Verification items for the finished model (mm, model axes). A direction names the side the tool comes from. Coordinates: 2 decimals unless noted, no trailing zeros. Write each loop counter-clockwise with the first axis right and the second up, starting at its lowest first coordinate (ties: lowest second). Pieces come first, ordered by that corner, then holes. Notation, with made-up numbers: (81, 38.25) -> (137, 38.25) arc R17 ccw to (137, 64.25) -> close; hole circle Ø7 at (8, 13). An arc over 180 degrees is marked (long way). Use a Markdown table: item, result. Add a question column.
from build123d import *

# Parameters (mm, degrees)
F0_R     = 14
F1_DEPTH = 40
F2_R     = 5.5
F3_DEPTH = 15
F2_R_2   = 9
F4_DEPTH = 7.3


with BuildPart() as f1:
    # F0 (on Front) → F1 (new body)
    with BuildSketch(Plane.XZ):
        with BuildLine():
            Line((-55, 0), (0, 0))
            Line((0, 0), (55, 0))
            Line((55, 0), (55, 15))
            Line((55, 15), (25, 15))
            Line((25, 15), (25, 40))
            ThreePointArc((25, 40), (0, 66), (-25, 40))
            Line((-25, 40), (-25, 15))
            Line((-25, 15), (-55, 15))
            Line((-55, 15), (-55, 0))
        make_face()
        with Locations((0, 40)):
            Circle(F0_R, mode=Mode.SUBTRACT)
    extrude(amount=F1_DEPTH)

    # F2 (on face) → F3 (cut)
    with BuildSketch(Plane.XY.offset(15)):
        with Locations((40, -20)):
            Circle(F2_R)
        with Locations((-40, -20)):
            Circle(F2_R)
    extrude(amount=-F3_DEPTH, mode=Mode.SUBTRACT)

    # F2 (on face) → F4 (cut)
    with BuildSketch(Plane.XY.offset(15)):
        with Locations((40, -20)):
            Circle(F2_R_2)
        with Locations((40, -20)):
            Circle(F2_R, mode=Mode.SUBTRACT)
        with Locations((-40, -20)):
            Circle(F2_R_2)
        with Locations((-40, -20)):
            Circle(F2_R, mode=Mode.SUBTRACT)
    extrude(amount=-F4_DEPTH, mode=Mode.SUBTRACT)


solid = f1.part
1) Thickness scan on L1, parallel to Y at x = 40, z = 11; L2, parallel to Y at x = 40, z = 2.75; L3, parallel to Z at x = -33.5, y = -20. Record the ranges inside material, lowest first.
2) Cross-section at B-B on x = 0. Record the boundary of the cut face in (y, z), then the cut area to 3 significant figures.
3) Cross-section at D-D on y = -32.5. Record the boundary of the cut face in (x, z).
4) Gauge pin test, flat ends, axial feed: pin 1 (14.5 mm diameter, centred on x = -40, y = -16.5, fed in from +Z); pin 2 (6.5 mm diameter, centred on x = -40, y = -20, fed in from -Z); pin 3 (20 mm diameter, centred on y = -20.5, z = 31, fed in from -X); pin 4 (1 mm diameter, centred on x = 8.5, y = -11.5, fed in from +Z). Record the tip position at first contact, or that the pin passes through.
5) Cross-section at A-A on y = -20. Record the boundary of the cut face in (x, z), then the cut area to 3 significant figures.
6) Release check for a two-part mould opening along Y. For faces 1 (the face through (34.505, -19.758, 3.904)), 2 (the face through (40.2, -10.8, 15)), 3 (the face through (-1, -40, 19)), 4 (the face through (-1, 0, 19)) record: released by +Y, released by -Y, zero draft, split by the parting line, or undercut.
7) Set-up check for faces 5 (the face through (44, -16, 7.7)), 6 (the face through (-1, -20, 0)): record each of +Z, -Z, +X, -X, +Y, -Y from which the full face is reachable in a straight line by a thin tool's end or side.
8) Cross-section at C-C on z = 30.5. Record the boundary of the cut face in (x, y), then the cut area to 3 significant figures.
Returned:
| question | item | result |
|---|---|---|
| 1 | L1 | y = -40 to -29, -11 to 0 |
| 1 | L2 | y = -40 to -25.5, -14.5 to 0 |
| 1 | L3 | z = 0 to 7.7 |
| 2 | outline | (-40, 0) -> (0, 0) -> (0, 26) -> (-40, 26) -> close; (-40, 54) -> (0, 54) -> (0, 66) -> (-40, 66) -> close |
| 2 | area | 1,520 mm² |
| 3 | outline | (-55, 0) -> (55, 0) -> (55, 15) -> (25, 15) -> (25, 40) arc R25.02 ccw (long way) to (-25, 40) -> (-25, 15) -> (-55, 15) -> close; hole circle Ø28 at (0, 40) |
| 4 | pin 1 | stops at z = 15 |
| 4 | pin 2 | passes through |
| 4 | pin 3 | stops at x = -25.02 |
| 4 | pin 4 | stops at z = 64.69 |
| 5 | outline | (-55, 0) -> (-45.5, 0) -> (-45.5, 7.7) -> (-49, 7.7) -> (-49, 15) -> (-55, 15) -> close; (-34.5, 0) -> (34.5, 0) -> (34.5, 7.7) -> (31, 7.7) -> (31, 15) -> (25, 15) -> (25, 40) arc R25.02 ccw (long way) to (-25, 40) -> (-25, 15) -> (-31, 15) -> (-31, 7.7) -> (-34.5, 7.7) -> close; (45.5, 0) -> (55, 0) -> (55, 15) -> (49, 15) -> (49, 7.7) -> (45.5, 7.7) -> close; hole circle Ø28 at (0, 40) |
| 5 | area | 2,880 mm² |
| 6 | face 1 | undercut |
| 6 | face 2 | zero draft |
| 6 | face 3 | released by -Y |
| 6 | face 4 | released by +Y |
| 7 | face 5 | +Z |
| 7 | face 6 | -Z, +X, -X, +Y, -Y |
| 8 | outline | (-25, -40) -> (-10.28, -40) -> (-10.28, 0) -> (-25, 0) -> close; (10.28, -40) -> (25, -40) -> (25, 0) -> (10.28, 0) -> close |
| 8 | area | 1,180 mm² |
